from build123d import *

# Parameters (mm, degrees)
SKETCH1_R           = 4.590078396
BOSS_EXTRUDE1_DEPTH = 6
SKETCH1_3_R         = 10
SKETCH1_3_R_2       = 4.590078396
BOSS_EXTRUDE2_DEPTH = 20
BOSS_EXTRUDE3_START = -5
BOSS_EXTRUDE3_DEPTH = 5


with BuildPart() as part:
    # Sketch1 → Boss-Extrude1 (new body)
    with BuildSketch(Plane(origin=(0, 0, 0), x_dir=(1, 0, 0), z_dir=(0, 1, 0))):
        with BuildLine():
            Line((38.176629583, -13.072793558), (30.598786144, 30.167258341))
            Line((30.598786144, 30.167258341), (30.598786144, 0))
            Line((30.598786144, 0), (-21.824717568, 0))
            Line((-21.824717568, 0), (22.829214597, -25.872426793))
            ThreePointArc((22.829214597, -25.872426793), (36.654329673, -26.84846253), (38.176629583, -13.072793558))
        make_face()
        with Locations(Location((30.24949737, -19.168740974, 0), (0, 0, 270))):
            Circle(SKETCH1_R, mode=Mode.SUBTRACT)
    extrude(amount=BOSS_EXTRUDE1_DEPTH)

    # Sketch1_3 → Boss-Extrude2 (add)
    # profile 1 of 2: a face of its own
    with BuildSketch(Plane(origin=(0, 0, 0), x_dir=(1, 0, 0), z_dir=(0, 1, 0))):
        with Locations((30.24949737, -19.168740974)):
            Circle(SKETCH1_3_R)
        with Locations(Location((30.24949737, -19.168740974, 0), (0, 0, 270))):
            Circle(SKETCH1_3_R_2, mode=Mode.SUBTRACT)
    # profile 2 of 2: a face of its own
    with BuildSketch(Plane(origin=(0, 0, 0), x_dir=(1, 0, 0), z_dir=(0, 1, 0))):
        with BuildLine():
            Line((38.176629583, -13.072793558), (30.598786144, 30.167258341))
            Line((30.598786144, 30.167258341), (30.598786144, 0))
            Line((30.598786144, 0), (20.24949737, 0))
            Line((20.24949737, 0), (20.24949737, -19.168740974))
            ThreePointArc((20.24949737, -19.168740974), (27.030128032, -9.701129815), (38.176629583, -13.072793558))
        make_face()
    extrude(amount=BOSS_EXTRUDE2_DEPTH)

    # Sketch2 → Boss-Extrude3 (add)
    with BuildSketch(Plane(origin=(0, 20, 0), x_dir=(1, 0, 0), z_dir=(0, 1, 0)).offset(BOSS_EXTRUDE3_START)):
        with BuildLine():
            ThreePointArc((22.829214597, -25.872426793), (20.916683547, -22.760201141), (20.24949737, -19.168740974))
            Line((20.24949737, -19.168740974), (20.24949737, -0.012610588))
            Line((20.24949737, -0.012610588), (-21.802952608, -0.012610588))
            Line((-21.802952608, -0.012610588), (22.829214597, -25.872426793))
        make_face()
    extrude(amount=BOSS_EXTRUDE3_DEPTH)


solid = part.part
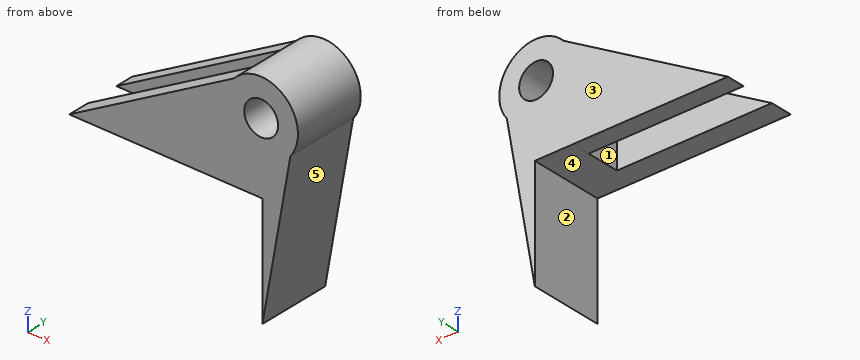
Source: CAD feature listing. Evaluate the final solid. Frame: model axes, mm. Face numbers are marked on the shaded views. A direction names the side the tool comes from. Coordinates: 2 decimals unless noted, no trailing zeros. Order: outer loops, then holes, each group sorted by start corner. A loop starts at its lowest first (then second) coordinate and runs counter-clockwise, first axis right, second up. Notation, with made-up numbers: M -39.5,45 L -5.5,45 A19 cw -5.5,58 Z; hole C -3,89.25 d8. An arc over 180 degrees is marked long. Write each question's results on one line, items separated by ' | '. Start each with the question number.
1. Section D-D, the plane z = 3. Return the cut outline in (x, y).
2. Draft query along Y for the marked faces 1, 2 and 3. Return one class per face: +Y half, -Y half, draft (parallel to the pull), parting line (faces both ways), or undercut.
3. Material intervals for L1, parallel to Y at x = 8, z = 16.5; L2, parallel to Z at x = 27, y = 10; L3, parallel to Z at x = 26, y = 12.5, sorted ascending.
4. Section B-B, the plane x = -9. Return the cut outline in (y, z), then the cut area to 3 significant figures.
5. Reachability of the marked faces 4 and 5 from +Z, -Z, +X, -X, +Y, -Y: full face, straight path, thin tool, end or side. Return the list, or none.
6. Pin query (flat end, axial travel): pin 1 (2.5 mm diameter, centred on x = -10.5, y = 18, fed in from -Z); pin 2 (3 mm diameter, centred on y = 2.5, z = 5, fed in from -X); pin 3 (5 mm diameter, centred on y = 13, z = -3, fed in from -X). Return the tip coordinate at first contact, or that it passes through.
7. Section A-A, the plane z = 22.5. Return the cut outline in (x, y).
Solution:
1) outline: M -16.65,0 L 36.41,0 L 36.41,20 L -16.65,20 L -16.65,15 L 20.25,15 L 20.25,6 L -16.65,6 Z
2) face 1: undercut | face 2: draft | face 3: +Y half
3) L1: 0 to 6, 15 to 20 | L2: 0 to 15.93, 22.41 to 28.63 | L3: 0 to 17.43, 20.9 to 28.22
4) outline: M 0,0 L 6,0 L 6,7.43 L 0,7.43 Z; M 15,0.01 L 20,0.01 L 20,7.43 L 15,7.43 Z | area: 81.7 mm²
5) face 4: -Z, -X, +Y, -Y | face 5: -Z, +X, +Y, -Y
6) pin 1: z = 0.01 | pin 2: x = -15.78 | pin 3: x = 30.6
7) outline: M 17.01,0 L 27.09,0 L 27.09,20 L 17.01,20 L 17.01,15 L 20.82,15 L 20.82,6 L 17.01,6 Z; M 33.41,0 L 39.68,0 L 39.68,20 L 33.41,20 Z
